from build123d import *

# Parameters (mm, degrees)
BOSS_EXTRUDE1_DEPTH    = 17.5
SKETCH1_3_R            = 16
SKETCH1_3_R_2          = 11
BOSS_EXTRUDE2_DEPTH    = 11
BOSS_EXTRUDE3_DEPTH    = 7.5
F_10_0MM_DOWEL_HOLE1_D = 10
FILLET1_RADIUS         = 7.5
FILLET1_LENGTH         = 22
FILLET2_RADIUS         = 7.5
FILLET2_LENGTH         = 22
CHAMFER1_SIZE          = 1.5
CHAMFER2_SIZE          = 1.5


with BuildPart() as part:
    # Sketch1 → Boss-Extrude1 (new, symmetric)
    with BuildSketch(Plane(origin=(0, 0, 0), x_dir=(1, 0, 0), z_dir=(0, 1, 0))):
        with BuildLine():
            Line((0, 31), (0, 25))
            ThreePointArc((0, 25), (25, 0), (0, -25))
            Line((0, -25), (0, -31))
            ThreePointArc((0, -31), (31, 0), (0, 31))
        make_face()
    extrude(amount=BOSS_EXTRUDE1_DEPTH, both=True)



with BuildPart() as body_2:
    # Sketch1<3> → Boss-Extrude2 (new, symmetric)
    with BuildSketch(Plane(origin=(0, 0, 0), x_dir=(1, 0, 0), z_dir=(0, 1, 0))):
        with Locations(Location((180, 0, 0), (0, 0, 270))):
            Circle(SKETCH1_3_R)
        with Locations(Location((180, 0, 0), (0, 0, 270))):
            Circle(SKETCH1_3_R_2, mode=Mode.SUBTRACT)
    extrude(amount=BOSS_EXTRUDE2_DEPTH, both=True)


with BuildPart() as part_1:
    add(part.part)

    add(body_2.part)  # Boss-Extrude3 merges body 2
    # Sketch1<4> → Boss-Extrude3 (add, symmetric)
    with BuildSketch(Plane(origin=(0, 0, 0), x_dir=(1, 0, 0), z_dir=(0, 1, 0))):
        with BuildLine():
            Line((0, 44.5), (0, 31))
            ThreePointArc((0, 31), (31, 0), (0, -31))
            Line((0, -31), (0, -44.5))
            Line((0, -44.5), (22, -44.5))
            Line((22, -44.5), (22, -36.368169362))
            ThreePointArc((22, -36.368169362), (36.913436466, -24.9211933), (55, -19.790884566))
            Line((55, -19.790884566), (159.279067997, -10.667648273))
            ThreePointArc((159.279067997, -10.667648273), (165.659496532, -11.136586007), (171.565414601, -13.596240993))
            ThreePointArc((171.565414601, -13.596240993), (164, 0), (171.565414601, 13.596240993))
            ThreePointArc((171.565414601, 13.596240993), (165.659496532, 11.136586007), (159.279067997, 10.667648273))
            Line((159.279067997, 10.667648273), (55, 19.790884566))
            ThreePointArc((55, 19.790884566), (36.913436466, 24.9211933), (22, 36.368169362))
            Line((22, 36.368169362), (22, 44.5))
            Line((22, 44.5), (0, 44.5))
        make_face()
        with BuildLine():
            ThreePointArc((56.282546806, -14.659577072), (40.284425725, 0), (56.282546806, 14.659577072))
            Line((56.282546806, 14.659577072), (155.522934456, 5.977168189))
            ThreePointArc((155.522934456, 5.977168189), (161, 0), (155.522934456, -5.977168189))
            Line((155.522934456, -5.977168189), (56.282546806, -14.659577072))
        make_face(mode=Mode.SUBTRACT)
    extrude(amount=BOSS_EXTRUDE3_DEPTH, both=True)

    # Ø10.0mm Dowel Hole1 (through all)
    with Locations(Plane.ZY):
        with Locations((-37, 0), (37, 0)):
            Hole(F_10_0MM_DOWEL_HOLE1_D / 2)

    # Fillet1: full round fillet: the end face becomes a half cylinder, R = half its width
    fillet1_face = Plane((11, 0, 44.5), x_dir=(1, 0, 0), z_dir=(0, 0, 1))  # on the end face: x along it, z out of the body
    fillet1_slab = fillet1_face.offset(-FILLET1_RADIUS / 2) * Box(FILLET1_LENGTH, 2 * FILLET1_RADIUS, FILLET1_RADIUS, mode=Mode.PRIVATE)  # the body's end, R deep
    fillet1_round = Plane((11, 0, 37), x_dir=(0, 0, 1), z_dir=(1, 0, 0)) * Cylinder(FILLET1_RADIUS, FILLET1_LENGTH, mode=Mode.PRIVATE)  # its axis R under the face
    add(fillet1_slab - fillet1_round, mode=Mode.SUBTRACT)

    # Fillet2: full round fillet: the end face becomes a half cylinder, R = half its width
    fillet2_face = Plane((11, 0, -44.5), x_dir=(1, 0, 0), z_dir=(0, 0, -1))  # on the end face: x along it, z out of the body
    fillet2_slab = fillet2_face.offset(-FILLET2_RADIUS / 2) * Box(FILLET2_LENGTH, 2 * FILLET2_RADIUS, FILLET2_RADIUS, mode=Mode.PRIVATE)  # the body's end, R deep
    fillet2_round = Plane((11, 0, -37), x_dir=(0, 0, -1), z_dir=(1, 0, 0)) * Cylinder(FILLET2_RADIUS, FILLET2_LENGTH, mode=Mode.PRIVATE)  # its axis R under the face
    add(fillet2_slab - fillet2_round, mode=Mode.SUBTRACT)

    # Chamfer1
    chamfer1_edges = [part_1.edges().sort_by_distance(p)[0] for p in [
        (105.902740631, -7.5, 10.31837263),
        (40.284425725, -7.5, 0),
        (105.902740631, -7.5, -10.31837263),
        (161, -7.5, 0),
        (105.902740631, 7.5, 10.31837263),
        (40.284425725, 7.5, 0),
        (105.902740631, 7.5, -10.31837263),
        (161, 7.5, 0),
    ]]
    chamfer(chamfer1_edges, length=CHAMFER1_SIZE)

    # Chamfer2
    chamfer2_edges = [part_1.edges().sort_by_distance(p)[0] for p in [
        (180, 11, -11),
        (180, -11, -11),
    ]]
    chamfer(chamfer2_edges, length=CHAMFER2_SIZE)


solid = part_1.part
Geometry: final body of the model. Coordinates: model frame, mm. A direction names the side the tool comes from. Give positions to 0.01 mm unless a question says otherwise; leave off trailing zeros. Loops run counter-clockwise (first coordinate to the right, second up) from the corner with the lowest first, then second, coordinate; pieces in that order, holes last. Notation, with made-up numbers: (28.5, -13.75) -> (56.5, -13.75) arc R23 cw to (56.5, -1.75) -> close; hole circle Ø11 at (55, 72.25). An arc over 180 degrees is marked (long way). Put each result on its own line as item: value.
1. Cut plane C-C (z = 0). Return the cut outline in (x, y).
Taken from the geometry:
outline: (25, -17.5) -> (31, -17.5) -> (31, -7.5) -> (38.78, -7.5) -> (40.28, -6) -> (40.28, 6) -> (38.78, 7.5) -> (31, 7.5) -> (31, 17.5) -> (25, 17.5) -> close; (161, -6) -> (162.5, -7.5) -> (164, -7.5) -> (164, -11) -> (167.5, -11) -> (169, -9.5) -> (169, 9.5) -> (167.5, 11) -> (164, 11) -> (164, 7.5) -> (162.5, 7.5) -> (161, 6) -> close; (191, -9.5) -> (192.5, -11) -> (196, -11) -> (196, 11) -> (192.5, 11) -> (191, 9.5) -> close
2. Set-up query: faces 1 (the flat face through (172, -11, -10)), 2 (the flat face through (106.664, -6.761, 11.015)), 3 (the flat face through (106.662, 6.739, 10.994)), 4 (the flat face through (107.869, 0.105, -15.165)). Return all of +Z, -Z, +X, -X, +Y, -Y with unobstructed straight access to the full face (end or side cutting, diameter ignored); none if empty.
Taken from the geometry:
face 1: +Z, -Z, +X, -Y
face 2: -Y
face 3: +Y
face 4: -Z, +Y, -Y
3. Pin query (flat end, axial travel): P1, Ø22, axis at x = 87, z = 17.5, coming from the +Y side; P2, Ø8, axis at y = 2, z = 8, coming from the +X side; P3, Ø6, axis at x = 43.5, y = -5.5, coming from the -Z side. Return the tip coordinate at first contact, or that it passes through.
Taken from the geometry:
P1: stops at y = 7.5
P2: stops at x = 195.49
P3: stops at z = -23.29
4. Cut plane B-B (x = 180). Return the cut outline in (y, z), plus the area to 4 significant figures.
Taken from the geometry:
outline: (-11, -16) -> (11, -16) -> (11, -12.5) -> (9.5, -11) -> (-9.5, -11) -> (-11, -12.5) -> close; (-11, 12.5) -> (-9.5, 11) -> (9.5, 11) -> (11, 12.5) -> (11, 16) -> (-11, 16) -> close
area: 215.5 mm2
5. Cut plane A-A (y = 0). Return the cut outline in (x, z).
Taken from the geometry:
outline: (0, -44.5) -> (22, -44.5) -> (22, -42) -> (0, -42) -> close; (0, -32) -> (26.4, -32) arc R50 cw to (55, -19.79) -> (159.28, -10.67) arc R20 cw to (171.57, -13.6) arc R16 ccw (long way) to (171.57, 13.6) arc R20 cw to (159.28, 10.67) -> (55, 19.79) arc R50 cw to (26.4, 32) -> (0, 32) -> (0, 25) arc R25 cw to (0, -25) -> close; (0, 42) -> (22, 42) -> (22, 44.5) -> (0, 44.5) -> close; hole (56.28, -14.66) -> (155.52, -5.98) arc R6 ccw to (155.52, 5.98) -> (56.28, 14.66) arc R14.72 ccw (long way) to start; hole circle Ø22 at (180, 0)
6. Cut plane D-D (z = -22.5). Return the cut outline in (x, y).
Taken from the geometry:
outline: (10.9, -17.5) -> (21.32, -17.5) -> (21.32, -7.5) -> (42.58, -7.5) -> (42.58, 7.5) -> (21.32, 7.5) -> (21.32, 17.5) -> (10.9, 17.5) -> close
7. Ray query, line 1 along X through (y, z) = (-5.5, 0); line 2 along Y through (x, z) = (18, 37); line 3 along X through (y, z) = (5, -3.5). Return the intervals inside material, ascending. Write a range as [from, to].
Taken from the geometry:
line 1: x = [25, 40.28], [161, 169], [191, 196]
line 2: y = [-7.5, -5], [5, 7.5]
line 3: x = [24.75, 40.71], [159.87, 169.57], [190.43, 195.61]
8. Pull-direction query (Z, two-part tool) for faces 5 (the flat face through (105.21, 0.08, -10.38)), 6 (the cylindrical face through (195.864, 0.154, -2.083)), 7 (the cylindrical face through (11.15, 0.16, 44.5)); classes: released by +Z, released by -Z, zero draft, split by the parting line, or undercut.
Taken from the geometry:
face 5: undercut
face 6: split by the parting line
face 7: released by +Z
